Source: CAD feature listing. Evaluate the final solid. Frame: model axes, mm. A direction names the side the tool comes from. Round coordinates to 2 decimals unless told otherwise and drop trailing zeros. Write each loop counter-clockwise with the first axis right and the second up, starting at its lowest first coordinate (ties: lowest second). Pieces come first, ordered by that corner, then holes.
```python
from build123d import *

# Parameters (mm, degrees)
PATTERN_CIRCULAR_1_COUNT = 2
PATTERN_CIRCULAR_1_ANGLE = 90


with BuildPart() as part:
    # 草图3 → Revolve 850 (revolve)
    with BuildSketch(Plane.XY, mode=Mode.PRIVATE) as revolve_850_sk:
        with BuildLine():
            Line((0, 0), (8, 0))
            Line((8, 0), (8, 1.5))
            Line((8, 1.5), (3, 1.5))
            Line((3, 1.5), (2.799, 1.299))
            Line((2.799, 1.299), (2.501, 1.299))
            ThreePointArc((2.501, 1.299), (2.146739503, 1.445739503), (2, 1.8))
            Line((2, 1.8), (2, 2.75))
            Line((2, 2.75), (0.182568851, 2.590995378))
            ThreePointArc((0.182568851, 2.590995378), (0.052544533, 2.52687448), (0, 2.391756438))
            Line((0, 2.391756438), (0, 0))
        make_face()
    revolve(revolve_850_sk.sketch.rotate(Axis((-2.16958059, 0, 0), (1, 0, 0)), 90), axis=Axis((-2.16958059, 0, 0), (1, 0, 0)))

    # 草图4 → 切除-旋转1 (revolve, cut)
    with BuildSketch(Plane.XY, mode=Mode.PRIVATE) as cut_revolve_1_sk:
        Polygon((7.752708003, 1.5), (8.252708003, 1.5), (8, 1.067), align=None)
    revolve(cut_revolve_1_sk.sketch.rotate(Axis((-0.21798541, 0, 0), (1, 0, 0)), 90), axis=Axis((-0.21798541, 0, 0), (1, 0, 0)), mode=Mode.SUBTRACT)

    # 草图5 → 切除-放样1 section 0
    with BuildSketch(Plane.ZY, mode=Mode.PRIVATE) as loft_1_s0:
        with BuildLine():
            Line((-0.25, 1.75), (0.25, 1.75))
            Line((0.25, 1.75), (0.25, -1.75))
            Line((0.25, -1.75), (-0.25, -1.75))
            Line((-0.25, -1.75), (-0.25, 1.75))
        make_face()
    loft_1 = loft([loft_1_s0.sketch, Vertex(0.86, 0, 0)], mode=Mode.SUBTRACT)

    # 阵列(圆周)1: 切除-放样1 ×2 about axis
    pattern_circular_1_axis = Axis((0, 0, 0), (1, 0, 0))
    for i in range(1, PATTERN_CIRCULAR_1_COUNT):
        add(loft_1.rotate(pattern_circular_1_axis, i * PATTERN_CIRCULAR_1_ANGLE / (PATTERN_CIRCULAR_1_COUNT - 1)), mode=Mode.SUBTRACT)


solid = part.part
```
Q1. Set-up query: faces 1 (the face through (8, 0, 0)), 2 (the face through (2, 1, -2)), 3 (the face through (0.24, -0.18, -0.67)). Return all of +Z, -Z, +X, -X, +Y, -Y with unobstructed straight access to the full face (end or side cutting, diameter ignored); none if empty.
Q2. Pin query (flat end, axial travel): P1, Ø1, axis at x = 7, z = -1.5, coming from the +Y side. Return the tip coordinate at first contact, or that it passes through.
Q3. Section query C-C, the plane x = 1.75. Output: boundary loops of the cut face in (y, z).
Q4. Line query: line 1 (X direction, y = -1.35, z = 1.95); line 2 (Z direction, x = 1, y = -2.05); line 3 (Y direction, x = 6.75, z = -0.2). Output: solid intervals per line, ascending.
Q5. Section query B-B, the plane x = 4. Output: boundary loops of the cut face in (y, z).
Q6. Section query A-A, the plane x = 0.75. Output: boundary loops of the cut face in (y, z).
Filled in:
1. face 1: +Z, -Z, +X, +Y, -Y
1. face 2: +X
1. face 3: -X
2. P1: stops at y = 1.12
3. outline: circle Ø5.46 at (0, 0)
4. line 1: x = 0 to 2
4. line 2: z = -1.7 to 1.7
4. line 3: y = -1.49 to 1.49
5. outline: circle Ø3 at (0, 0)
6. outline: circle Ø5.28 at (0, 0); hole (-0.22, -0.03) - (-0.03, -0.03) - (-0.03, -0.22) - (0.03, -0.22) - (0.03, -0.03) - (0.22, -0.03) - (0.22, 0.03) - (0.03, 0.03) - (0.03, 0.22) - (-0.03, 0.22) - (-0.03, 0.03) - (-0.22, 0.03) - close
